Check sheet for the modelled part. Datum: model origin and axes. Units: mm. A direction names the side the tool comes from. Round coordinates to 2 decimals unless told otherwise and drop trailing zeros. Write each loop counter-clockwise with the first axis right and the second up, starting at its lowest first coordinate (ties: lowest second). Pieces come first, ordered by that corner, then holes. Notation, with made-up numbers: (50.5, -7) - (109.5, -7) arc R26 cw to (109.5, 12) - close; hole circle Ø6 at (47, -12.75). An arc over 180 degrees is marked (long way). Use one line per item in the form item = value. Start each with the question number.
1) Section check C-C (y = -2.5). Record the boundary of the cut face in (x, z), then the cut area to 3 significant figures.
2) Draft check along Z on faces 4 (the face through (-0.9, -6.9, -0.93)), 5 (the face through (5, 0, -1)), 6 (the face through (-0.8, 0, 7.8)), 7 (the face through (-1, -7, 10)). Enter one of: +Z half, -Z half, draft (parallel to the pull), parting line (faces both ways), or undercut.
3) Section check B-B (x = 6). Record the boundary of the cut face in (y, z).
4) Set-up check for faces 1 (the face through (0, -7, 3)), 2 (the face through (8, -9, 0)), 3 (the face through (-0.8, -14, 3.2)): record each of +Z, -Z, +X, -X, +Y, -Y from which the full face is reachable in a straight line by a thin tool's end or side.
5) Section check A-A (y = -7). Record the boundary of the cut face in (x, z).
6) Section check D-D (x = 10). Record the boundary of the cut face in (y, z).
7) Gauge pin test, flat ends, axial feed: P1, Ø4, axis at x = 8.5, y = 0, coming from the +Z side; P2, Ø0.8, axis at x = 3.5, z = -0.5, coming from the -Y side; P3, Ø2, axis at y = -13, z = 2.5, coming from the +X side; P4, Ø4.5, axis at x = 14, z = 4, coming from the +Y side. Record the tip position at first contact, or that the pin passes through.
8) Scan lines: probe 1 along X at (y, z) = (-5.25, 3); probe 2 along Y at (x, z) = (-1.2, 6); probe 3 along X at (y, z) = (-10.75, 0.5). Record each from-to range of solid material in increasing order.
from build123d import *

# Parameters (mm, degrees)
SKETCH_1_W             = 11
SKETCH_1_H             = 14
SM_BASE_FLANGE_1_DEPTH = 1.5
SKETCH_9_R             = 4.5
SKETCH_9_R_2           = 3
EXTRUDE_1_DEPTH        = 15
SKETCH_10_W            = 1.5
SKETCH_10_H            = 14
EXTRUDE_1_2_DEPTH      = 4.5
SKETCH_11_W            = 1.5
SKETCH_11_H            = 14
EXTRUDE_2_DEPTH        = 11.5
FILLET_2_R             = 2
FILLET_3_R             = 1
SKETCH_12_W            = 9
SKETCH_12_H            = 3.5
EXTRUDE_3_DEPTH        = 1.5
FILLET_4_R             = 2
SKETCH_13_R            = 1.8
CUT_EXTRUDE_1_DEPTH    = 1.5
SKETCH_14_R            = 2.076590198
CUT_EXTRUDE_2_DEPTH    = 1.5


# Sheet-metal steps are written as plain solids
with BuildPart() as part:
    # Sketch 1 → Базовая кромка1 (new body)
    with BuildSketch(Plane.XY):
        with Locations((5.5, -7)):
            Rectangle(SKETCH_1_W, SKETCH_1_H)
    extrude(amount=-SM_BASE_FLANGE_1_DEPTH)



with BuildPart() as body_2:
    # Эскиз9 → Extrude 1 (new body)
    with BuildSketch(Plane(origin=(0, -14.5, 0), x_dir=(-1, 0, 0), z_dir=(0, -1, 0))):
        with Locations((-15.5, -3)):
            Circle(SKETCH_9_R)
        with Locations((-15.5, -3)):
            Circle(SKETCH_9_R_2, mode=Mode.SUBTRACT)
    extrude(amount=-EXTRUDE_1_DEPTH)


with BuildPart() as part_1:
    add(part.part)

    add(body_2.part)  # Extrude 1 2 merges body 2
    # Эскиз10 → Extrude 1 2 (add)
    with BuildSketch(Plane(origin=(11, 0, 0), x_dir=(0, 0, -1), z_dir=(1, 0, 0))):
        with Locations((0.75, -7)):
            Rectangle(SKETCH_10_W, SKETCH_10_H)
    extrude(amount=EXTRUDE_1_2_DEPTH)

    # Эскиз11 → Бобышка-Вытянуть2 (add)
    with BuildSketch(Plane(origin=(0, 0, -1.5), x_dir=(-1, 0, 0), z_dir=(0, 0, -1))):
        with Locations((0.75, -7)):
            Rectangle(SKETCH_11_W, SKETCH_11_H)
    extrude(amount=-EXTRUDE_2_DEPTH)

    # Скругление2
    fillet_2_edges = [part_1.edges().sort_by_distance(p)[0] for p in [
        (-1.5, -7, -1.5),
    ]]
    fillet(fillet_2_edges, radius=FILLET_2_R)

    # Скругление3
    fillet_3_edges = [part_1.edges().sort_by_distance(p)[0] for p in [
        (0, -7, 0),
    ]]
    fillet(fillet_3_edges, radius=FILLET_3_R)

    # Эскиз12 → Бобышка-Вытянуть3 (add)
    with BuildSketch(Plane.ZY.offset(1.5)):
        with Locations((5.5, -15.75)):
            Rectangle(SKETCH_12_W, SKETCH_12_H)
        with Locations((5.5, 1.75)):
            Rectangle(SKETCH_12_W, SKETCH_12_H)
    extrude(amount=-EXTRUDE_3_DEPTH)

    # Скругление4
    fillet_4_edges = [part_1.edges().sort_by_distance(p)[0] for p in [
        (-0.75, -17.5, 10),
        (-0.75, -17.5, 1),
        (-0.75, 3.5, 10),
        (-0.75, 3.5, 1),
    ]]
    fillet(fillet_4_edges, radius=FILLET_4_R)

    # Эскиз13 → Вырез-Вытянуть1 (cut)
    with BuildSketch(Plane.ZY.offset(1.5)):
        with Locations((6, -7)):
            Circle(SKETCH_13_R)
        with BuildLine():
            Line((5, 1.8), (6, 1.8))
            ThreePointArc((6, 1.8), (7.8, 0), (6, -1.8))
            Line((6, -1.8), (5, -1.8))
            ThreePointArc((5, -1.8), (3.2, 0), (5, 1.8))
        make_face()
        with BuildLine():
            Line((5, -15.8), (6, -15.8))
            ThreePointArc((6, -15.8), (7.8, -14), (6, -12.2))
            Line((6, -12.2), (5, -12.2))
            ThreePointArc((5, -12.2), (3.2, -14), (5, -15.8))
        make_face()
    extrude(amount=-CUT_EXTRUDE_1_DEPTH, mode=Mode.SUBTRACT)

    # Эскиз14 → Вырез-Вытянуть2 (cut)
    with BuildSketch(Plane(origin=(0, 0, -1.5), x_dir=(-1, 0, 0), z_dir=(0, 0, -1))):
        with Locations((-6, -7)):
            Circle(SKETCH_14_R)
    extrude(amount=-CUT_EXTRUDE_2_DEPTH, mode=Mode.SUBTRACT)


solid = part_1.part
Results are:
q1.outline = (-1.5, 0.5) arc R2 ccw to (0.5, -1.5) - (15.5, -1.5) arc R4.5 ccw (long way) to (12.15, 0) - (1, 0) arc R1 cw to (0, 1) - (0, 10) - (-1.5, 10) - close; hole circle Ø6 at (15.5, 3)
q1.area = 71.7 mm²
q2.face_4 = -Z half
q2.face_5 = draft
q2.face_6 = undercut
q2.face_7 = +Z half
q3.outline = (-14, -1.5) - (-9.08, -1.5) - (-9.08, 0) - (-14, 0) - close; (-4.92, -1.5) - (0, -1.5) - (0, 0) - (-4.92, 0) - close
q4.face_1 = +Z, +Y, -Y
q4.face_2 = +Y, -Y
q4.face_3 = -X
q5.outline = (-1.5, 0.5) arc R2 ccw to (0.5, -1.5) - (3.92, -1.5) - (3.92, 0) - (1, 0) arc R1 cw to (0, 1) - (0, 4.2) - (-1.5, 4.2) - close; (-1.5, 7.8) - (0, 7.8) - (0, 10) - (-1.5, 10) - close; (8.08, -1.5) - (15.5, -1.5) arc R4.5 ccw (long way) to (12.15, 0) - (8.08, 0) - close; hole circle Ø6 at (15.5, 3)
q6.outline = (-14, -1.5) - (0, -1.5) - (0, 0) - (-14, 0) - close
q7.P1 = 0
q7.P2 = -14
q7.P3 = 20
q7.P4 = 0.5
q8.probe_1 = -1.5 to 0, 11 to 12.5, 18.5 to 20
q8.probe_2 = -17.5 to -15.8, -12.2 to -8.8, -5.2 to -1.8, 1.8 to 3.5
q8.probe_3 = -1.5 to 0.13, 11.76 to 13.84, 17.16 to 19.24
